The listing builds one solid part. Answer for the finished solid, in the listing's coordinates (mm). Round coordinates to 2 decimals unless told otherwise and drop trailing zeros. Write each loop counter-clockwise with the first axis right and the second up, starting at its lowest first coordinate (ties: lowest second). Pieces come first, ordered by that corner, then holes. Notation, with made-up numbers: M -40,39.5 L -20,39.5 A18 cw -20,70.5 Z; hole C 61,65 d5. An arc over 180 degrees is marked long. One line per item, written item: value. Start each with the question number.
(1) Given P1, Ø3, axis at x = 97, z = -2.5, coming from the -Y side; P2, Ø1, axis at x = -93.5, z = -4, coming from the +Y side; P3, Ø3, axis at x = 45, y = 124, coming from the -Z side, each flat-ended and moving along its own axis, determine where each tip first touches the part or whether it passes through.
(2) Consider probe 1 along Z at (x, y) = (-168.5, 71); probe 2 along X at (y, z) = (-7, -5); probe 3 along X at (y, z) = (-55.5, -4.75). Determine where each line is inside the solid, lowest interval first.
(3) Section C-C (z = -1.25) is taken. Determine the outline of the cut face in (x, y) (3 decimals).
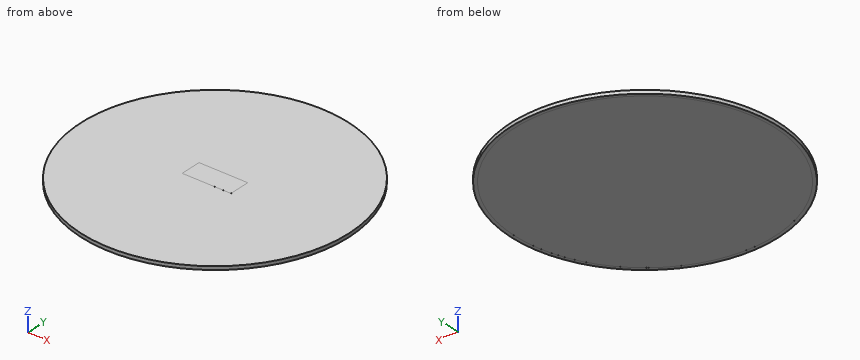
```python
from build123d import *

# Parameters (mm, degrees)
F2_W     = 88.9
F2_H     = 38.1
F3_DEPTH = 0.0254


with BuildPart() as f1:
    # F0 (on Front) → F1 (revolve)
    with BuildSketch(Plane.XZ):
        Polygon((244.475, 0), (0, 0), (0, -6.35), (238.125, -6.35), (238.125, -6.3754), (244.475, -6.3754), align=None)
    revolve(axis=Axis((0, 0, -42.829115), (0, 0, -1)))

    # F2 (on face) → F3 (join)
    with BuildSketch(Plane.XY):
        Rectangle(F2_W, F2_H)
    extrude(amount=F3_DEPTH)


solid = f1.part
```
Recorded:
1. P1: stops at y = -225.05
1. P2: stops at y = 226.1
1. P3: stops at z = -6.35
2. probe 1: z = -6.35 to 0
2. probe 2: x = -244.37 to 244.37
2. probe 3: x = -238.09 to 238.09
3. outline: C 0,0 d488.95
